Autodesk Inventor part; units mm, degrees
ref_plane "YZ Plane" through (0, 0, 0) normal (1, 0, 0) x (0, 1, 0)
ref_plane "XZ Plane" through (0, 0, 0) normal (0, 1, 0) x (-1, 0, 0)
ref_plane "XY Plane" through (0, 0, 0) normal (0, 0, 1) x (1, 0, 0)
sketch "Boceto1" plane through (0, 0, 0) normal (0, 1, 0) x (-1, 0, 0)
  line L0 (0, 0) -> (100, 0)
  line L1 (100, 0) -> (100, -130)
  line L2 (100, -130) -> (0, -130)
  line L3 (0, -130) -> (0, 0)
  dimension "d0" = 100
  dimension "d1" = 130
extrude "Extrusión1" add sketch "Boceto1" along normal blind 28
sketch "Boceto2" plane through (0, 28, 0) normal (0, 1, 0) x (1, 0, 0)
  line L0 (-70, 13.56) -> (-30, 13.56)
  line L1 (-30, 13.56) -> (-30, 14.36)
  line L2 (-30, 14.36) -> (-70, 14.36)
  line L3 (-70, 14.36) -> (-70, 13.56)
  line L4 (-100, 0) -> (0, 0)
  line L5 (0, 0) -> (0, 130)
  line L6 (-70, 16.36) -> (-30, 16.36)
  line L7 (-30, 16.36) -> (-30, 17.26)
  line L8 (-30, 17.26) -> (-70, 17.26)
  line L9 (-70, 17.26) -> (-70, 16.36)
  line L10 (-70, 19.26) -> (-30, 19.26)
  line L11 (-30, 19.26) -> (-30, 20.16)
  line L12 (-30, 20.16) -> (-70, 20.16)
  line L13 (-70, 20.16) -> (-70, 19.26)
  line L14 (-85, 85) -> (-15, 85)
  line L15 (-15, 85) -> (-15, 35)
  line L16 (-15, 35) -> (-85, 35)
  line L17 (-85, 35) -> (-85, 85)
  line L18 (-100, 130) -> (-100, 0)
  line L19 (0, 130) -> (-100, 130)
  circle A0 centre (-50, 107.5) radius 4.5
  dimension "d4" = 40
  dimension "d5" = 0.8
  dimension "d6" = 13.56
  dimension "d7" = 30
  dimension "d8" = 40
  dimension "d9" = 0.9
  dimension "d10" = 2
  dimension "d11" = 0
  dimension "d12" = 40
  dimension "d13" = 0.9
  dimension "d14" = 0
  dimension "d15" = 2
  dimension "d16" = 70
  dimension "d17" = 50
  dimension "d18" = 15
  dimension "d19" = 45
  dimension "d20" = 9
  dimension "d21" = 50
  dimension "d22" = 22.5
extrude "Extrusión2" cut sketch "Boceto2" against normal blind 28 contours L3 L2 L1 L0 | L9 L8 L7 L6 | L13 L12 L11 L10 | L14 L15 L16 L17 | A0
sketch "Boceto3" plane through (-100, 0, -130) normal (-1, 0, 0) x (0, 0, 1)
  line L0 (95, 0) -> (45, 0)
  arc A0 (56.5512, 0) -> (46.5113, 0) centre (51.5312, -0.2684) ccw
  point P0 (130, 0)
extrude "Extrusión3" cut sketch "Boceto3" against normal blind 15
equation "\"Radio_pliegue\" = Grosor"
equation "\"Anchura_desahogo_plegado\" = Grosor"
equation "\"Profundidad_desahogo_plegado\" = 0.5 * Grosor"
equation "\"Tamaño_destalonado\" = 4 * Grosor"
equation "\"Remanente_mínimo\" = 2 * Grosor"
equation "\"Radiodetransición\" = Radio_pliegue"
equation "\"Tamaño_de_radio_de_Jacobi\" = Radio_pliegue"
equation "\"TamañoSeparación\" = Grosor"
properties part number "carcasaV2"
Could you check a few things on this model? Use its own coordinates, in mm. A direction names the side the tool comes from. Coordinates: 2 decimals unless noted, no trailing zeros. Write each loop counter-clockwise with the first axis right and the second up, starting at its lowest first coordinate (ties: lowest second). Pieces come first, ordered by that corner, then holes. Notation, with made-up numbers: (12.25, -4) -> (36.25, -4) arc R23 cw to (36.25, 6) -> close; hole circle Ø3 at (-21.75, -18.75). An arc over 180 degrees is marked (long way). Write item = value, one per line. Start each with the question number.
(1) Which directions (+Z, -Z, +X, -X, +Y, -Y) give clear straight access to the entire face, cutting with the end or side of a thin tool? Please do faces 1 (the face through (-49, 0, -93)), 2 (the face through (-50, 14, -20.16)).
(2) I want a section at C-C (x = -50). Please give me the cut outline in (y, z).
(3) I want a section at B-B (z = -107.5). Please give me the cut outline in (x, y), plus the area to 3 significant figures.
(4) I need wall thicknesses on line 1 (Z direction, x = -50, y = 5.75); line 2 (Z direction, x = -30.5, y = 17.5); line 3 (X direction, y = 9.75, z = -107.5). Which ranges of each line are inside material? Lowest first, please. Write a range as [from, to].
(5) I want a section at A-A (x = -71.5). Please give me the cut outline in (y, z).
(6) We'd pull the mould along X, two halves only. Please class faces 3 (the face through (-92.605, 4.758, -78.362)), 4 (the face through (-100, 14, -64)), 5 (the face through (-85, 14, -60)): released by +X, released by -X, zero draft, split by the parting line, or undercut.
(7) Will this pin go through, and if not, where does the flat tip stop? pin 1 (7 mm diameter, centred on x = -50, z = -107.5, fed in from -Y) (3 decimals).
(8) I want a section at D-D (y = 12.5). Please give me the cut outline in (x, z), plus the area to 3 significant figures.
Result set:
q1.face_1 = +Z, -Z, +X, -X, -Y
q1.face_2 = +Y, -Y
q2.outline = (0, -130) -> (28, -130) -> (28, -112) -> (0, -112) -> close; (0, -103) -> (28, -103) -> (28, -85) -> (0, -85) -> close; (0, -35) -> (28, -35) -> (28, -20.16) -> (0, -20.16) -> close; (0, -19.26) -> (28, -19.26) -> (28, -17.26) -> (0, -17.26) -> close; (0, -16.36) -> (28, -16.36) -> (28, -14.36) -> (0, -14.36) -> close; (0, -13.56) -> (28, -13.56) -> (28, 0) -> (0, 0) -> close
q3.outline = (-100, 0) -> (-54.5, 0) -> (-54.5, 28) -> (-100, 28) -> close; (-45.5, 0) -> (0, 0) -> (0, 28) -> (-45.5, 28) -> close
q3.area = 2,550 mm2
q4.line_1 = [-130, -112], [-103, -85], [-35, -20.16], [-19.26, -17.26], [-16.36, -14.36], [-13.56, 0]
q4.line_2 = [-130, -85], [-35, -20.16], [-19.26, -17.26], [-16.36, -14.36], [-13.56, 0]
q4.line_3 = [-100, -54.5], [-45.5, 0]
q5.outline = (0, -130) -> (28, -130) -> (28, -85) -> (0, -85) -> close; (0, -35) -> (28, -35) -> (28, 0) -> (0, 0) -> close
q6.face_3 = zero draft
q6.face_4 = released by -X
q6.face_5 = undercut
q7.pin_1 = through
q8.outline = (-100, -130) -> (0, -130) -> (0, 0) -> (-100, 0) -> close; hole (-85, -85) -> (-15, -85) -> (-15, -35) -> (-85, -35) -> close; hole (-70, -20.16) -> (-30, -20.16) -> (-30, -19.26) -> (-70, -19.26) -> close; hole (-70, -17.26) -> (-30, -17.26) -> (-30, -16.36) -> (-70, -16.36) -> close; hole (-70, -14.36) -> (-30, -14.36) -> (-30, -13.56) -> (-70, -13.56) -> close; hole circle Ø9 at (-50, -107.5)
q8.area = 9,330 mm2
